from build123d import *

# Parameters (mm, degrees)
F0_R     = 12
F0_R_2   = 8
F1_DEPTH = 8
F2_R     = 1
F3_R     = 2
F4_DEPTH = 30


with BuildPart() as f1:
    # F0 (on Top) → F1 (new body)
    with BuildSketch(Plane.XY):
        Circle(F0_R)
        Circle(F0_R_2, mode=Mode.SUBTRACT)
    extrude(amount=F1_DEPTH)

    # F2
    f2_edges = [f1.edges().sort_by_distance(p)[0] for p in [
        (-12, 0, 8),
    ]]
    fillet(f2_edges, radius=F2_R)

    # F3 (on Right) → F4 (cut, symmetric)
    with BuildSketch(Plane.YZ):
        with Locations((0, 4)):
            Circle(F3_R)
    extrude(amount=F4_DEPTH, both=True, mode=Mode.SUBTRACT)


solid = f1.part
Verification items for the finished model (mm, model axes). Coordinates: 2 decimals unless noted, no trailing zeros. Order: outer loops, then holes, each group sorted by start corner. A loop starts at its lowest first (then second) coordinate and runs counter-clockwise, first axis right, second up. Notation, with made-up numbers: M -14,61.25 L 34,61.25 A15 ccw 34,84.25 Z; hole C 30,-6 d10. An arc over 180 degrees is marked long. One line per item, written item: value. Start each with the question number.
Item 1: Depth check by flat-ended pin: P1, Ø4, axis at x = -4.5, z = 1.5, coming from the -Y side; P2, Ø1, axis at x = -4, z = 5.5, coming from the +Y side; P3, Ø1.5, axis at y = -1.5, z = 5, coming from the +X side. Enter the tip coordinate at first touch or a pass-through.
Item 2: Sectioned sample at C-C on z = 5.25. Record the cut outline in (x, y).
Item 3: Sectioned sample at B-B on x = 0. Record the cut outline in (y, z), then the cut area to 3 significant figures.
Item 4: Thickness scan on probe 1 along Y at (x, z) = (0, 5); probe 2 along Z at (x, y) = (9.7, 0); probe 3 along Y at (x, z) = (9.85, 4). Record the ranges inside material, lowest first.
Item 5: Sectioned sample at A-A on y = 0. Record the cut outline in (x, z).
Item 6: Sectioned sample at D-D on z = 0.75. Record the cut outline in (x, y).
Item 7: Mould release check, pull along Y, two halves, no side actions. Record for faces 1 (the cylindrical face through (-9.842, 1.847, 3.234)), 2 (the flat face through (-2, -8, 8)), 3 (the cylindrical face through (11.446, 3.604, 3.451)), 4 (the cylindrical face through (10, 0, 2)): pulls with the +Y half, pulls with the -Y half, needs draft (parallel to the pull), parting line crosses it, or undercut.
Calculated:
1. P1: y = -11.74
1. P2: y = 11.48
1. P3: x = 11.95
2. outline: M -11.9,-1.56 A12 ccw 11.9,-1.56 L 7.85,-1.56 A8 cw -7.85,-1.56 Z; M -11.9,1.56 L -7.85,1.56 A8 cw 7.85,1.56 L 11.9,1.56 A12 ccw Z
3. outline: M -12,0 L -8,0 L -8,8 L -11,8 A1 ccw -12,7 Z; M 8,0 L 12,0 L 12,7 A1 ccw 11,8 L 8,8 Z
3. area: 63.6 mm^2
4. probe 1: -12 to -8, 8 to 12
4. probe 2: 0 to 2, 6 to 8
4. probe 3: -6.85 to -2, 2 to 6.85
5. outline: M -12,0 L -8,0 L -8,2 L -12,2 Z; M -12,6 L -8,6 L -8,8 L -11,8 A1 ccw -12,7 Z; M 8,0 L 12,0 L 12,2 L 8,2 Z; M 8,6 L 12,6 L 12,7 A1 ccw 11,8 L 8,8 Z
6. outline: C 0,0 d24; hole C 0,0 d16
7. face 1: undercut
7. face 2: needs draft
7. face 3: parting line crosses it
7. face 4: undercut
